Source: CAD feature listing. Evaluate the final solid. Frame: model axes, mm. Face numbers are marked on the shaded views. A direction names the side the tool comes from. Give positions to 0.01 mm unless a question says otherwise; leave off trailing zeros. Write each loop counter-clockwise with the first axis right and the second up, starting at its lowest first coordinate (ties: lowest second). Pieces come first, ordered by that corner, then holes. Notation, with made-up numbers: (70.5, 36) -> (103.5, 36) arc R30 ccw to (103.5, 66) -> close; hole circle Ø4 at (68.5, 35.25). An arc over 180 degrees is marked (long way). Answer as a JSON object with one key per item and string values. Group by question number.
Item 1: Access query for the marked faces 5, 6 and 7. Directions: +Z, -Z, +X, -X, +Y, -Y. A direction counts if a zero-diameter tool reaches every point of the face in a straight line with its end or side. Return the directions, or none.
Item 2: First-contact query: pin 1 Ø5 at (y, z) = (-3.5, 8) entering from -X; pin 2 Ø3 at (y, z) = (2.5, 10.5) entering from +X; pin 3 Ø3.5 at (x, z) = (13, 10.5) entering from -Y. Flat tips, straight axial feed; report the tip coordinate or a pass-through.
Item 3: Pull-direction query (X, two-part tool) for the marked faces 1, 2, 3 and 4; classes: pulls with the +X half, pulls with the -X half, needs draft (parallel to the pull), parting line crosses it, or undercut.
Item 4: Section query A-A on x = -15. Return the cut outline in (y, z).
Item 5: Section query D-D on y = 10. Return the cut outline in (x, z).
Item 6: Section query C-C on y = 3.5. Return the cut outline in (x, z).
Item 7: Ray query, probe 1 along Z at (x, y) = (-15, 9.5); probe 2 along X at (y, z) = (0, 7.75); probe 3 along Y at (x, z) = (0, 4.75). Return the intervals inside material, ascending. Write a range as from..to.
Item 8: Section query B-B on z = 8. Return the cut outline in (x, y), plus the area to 3 significant figures.
from build123d import *

# Parameters (mm, degrees)
ESBO_O1_R                = 7
RESSALTO_EXTRUS_O1_DEPTH = 16
ESBO_O2_W                = 1
ESBO_O2_H                = 5.647679103
CORTE_EXTRUS_O1_DEPTH    = 17
ESBO_O3_R                = 1.5
CORTE_EXTRUS_O2_DEPTH    = 16


with BuildPart() as part:
    # Esboço1 → Ressalto-extrusão1 (new body)
    with BuildSketch(Plane.XY):
        Polygon((-20, 8), (-8.5, 8), (-8.5, -10), (8.5, -10), (8.5, 8), (20, 8), (20, 13), (-20, 13), align=None)
        Circle(ESBO_O1_R, mode=Mode.SUBTRACT)
    extrude(amount=RESSALTO_EXTRUS_O1_DEPTH)

    # Esboço2 → Corte-extrusão1 (cut, through all)
    with BuildSketch(Plane.XY.offset(16)):
        with Locations((-0.048670763, -9.044181363)):
            Rectangle(ESBO_O2_W, ESBO_O2_H)
    extrude(amount=-CORTE_EXTRUS_O1_DEPTH, mode=Mode.SUBTRACT)

    # Esboço3 → Corte-extrusão2 (cut)
    with BuildSketch(Plane.XZ.offset(-8)):
        with Locations((-15, 8)):
            Circle(ESBO_O3_R)
    corte_extrus_o2 = extrude(amount=-CORTE_EXTRUS_O2_DEPTH, mode=Mode.SUBTRACT)

    # Espelhar1: Corte-extrusão2 across plane
    add(corte_extrus_o2.mirror(Plane(origin=(0, 0, 0), x_dir=(0, 0, 1), z_dir=(1, 0, 0))), mode=Mode.SUBTRACT)


solid = part.part
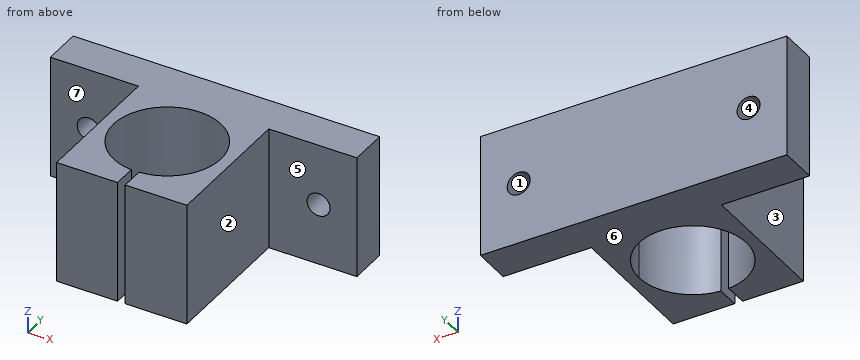
Worked answers:
{
 "1": {"face 5": "+Z, -Z, +X, -Y", "face 6": "-Z, +X, -X, +Y, -Y", "face 7": "+Z, -Z, -X, -Y"},
 "2": {"pin 1": "x = -8.5", "pin 2": "x = 8.5", "pin 3": "y = 8"},
 "3": {"face 1": "undercut", "face 2": "pulls with the +X half", "face 3": "pulls with the -X half", "face 4": "undercut"},
 "4": {"outline": "(8, 0) -> (13, 0) -> (13, 6.5) -> (8, 6.5) -> close; (8, 9.5) -> (13, 9.5) -> (13, 16) -> (8, 16) -> close"},
 "5": {"outline": "(-20, 0) -> (20, 0) -> (20, 16) -> (-20, 16) -> close; hole circle Ø3 at (-15, 8); hole circle Ø3 at (15, 8)"},
 "6": {"outline": "(-8.5, 0) -> (-6.06, 0) -> (-6.06, 16) -> (-8.5, 16) -> close; (6.06, 0) -> (8.5, 0) -> (8.5, 16) -> (6.06, 16) -> close"},
 "7": {"probe 1": "0..6.5, 9.5..16", "probe 2": "-8.5..-7, 7..8.5", "probe 3": "7..13"},
 "8": {"outline": "(-20, 8) -> (-16.5, 8) -> (-16.5, 13) -> (-20, 13) -> close; (-13.5, 8) -> (-8.5, 8) -> (-8.5, -10) -> (-0.55, -10) -> (-0.55, -6.98) arc R7 cw (long way) to (0.45, -6.99) -> (0.45, -10) -> (8.5, -10) -> (8.5, 8) -> (13.5, 8) -> (13.5, 13) -> (-13.5, 13) -> close; (16.5, 8) -> (20, 8) -> (20, 13) -> (16.5, 13) -> close", "area": "319 mm^2"}
}
